```python
from build123d import *

# Parameters (mm, degrees)
F0_R     = 43.2404063775
F1_DEPTH = 77
F1_TAPER = 3
F2_R     = 5
F3_T     = 2.5


with BuildPart() as f1:
    # F0 (on Top) → F1 (new body)
    with BuildSketch(Plane.XY):
        Circle(F0_R)
    extrude(amount=-F1_DEPTH, taper=F1_TAPER)

    # F2
    f2_edges = [f1.edges().sort_by_distance(p)[0] for p in [
        (-39.205007, 0, -77),
    ]]
    fillet(f2_edges, radius=F2_R)

    # F3
    f3_openings = [f1.faces().sort_by_distance(p)[0] for p in [
        (0, 0, 0),
    ]]
    offset(amount=F3_T, openings=f3_openings, kind=Kind.INTERSECTION)


solid = f1.part
```
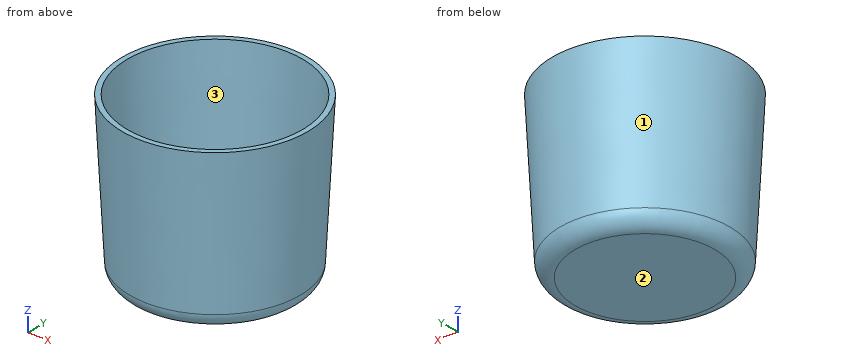
Design review of the part built by this model. Coordinates are the model's own, in mm. Face numbers are marked on the shaded views. Give positions to 0.01 mm unless a question says otherwise; leave off trailing zeros. Loops run counter-clockwise (first coordinate to the right, second up) from the corner with the lowest first, then second, coordinate; pieces in that order, holes last. Notation, with made-up numbers: (-21.5, 62.25) -> (-8.5, 62.25) arc R26 ccw to (-8.5, 92.25) -> close; hole circle Ø6 at (82.25, 81.5). An arc over 180 degrees is marked (long way). One line per item, written item: value.
Q1. For L1, parallel to Z at x = -21.5, y = -22.5; L2, parallel to X at y = -29.5, z = -13; L3, parallel to X at y = -31.5, z = -61.5, list the stretches that pass through material, from the lowest coordinate up.
Numbers:
L1: z = -79.5 to -77
L2: x = -34.06 to -30.68, 30.68 to 34.06
L3: x = -28.56 to -24.68, 24.68 to 28.56
Q2. We need section B-B on z = -52.5. Give the boundary of the cut face in (x, y).
Numbers:
outline: circle Ø85.98 at (0, 0); hole circle Ø80.98 at (0, 0)
Q3. For pin 1 Ø10 at (x, y) = (24.5, 21.5) entering from +Z; pin 2 Ø3 at (y, z) = (-28.5, -54.5) entering from +X; pin 3 Ø1.5 at (x, y) = (19, -10) entering from +Z, all flat-tipped, find the tip position at first contact; note any pin that passes through.
Numbers:
pin 1: stops at z = -75.89
pin 2: stops at x = 33.33
pin 3: stops at z = -77
Q4. We need section C-C on z = -38. Give the boundary of the cut face in (x, y).
Numbers:
outline: circle Ø87.5 at (0, 0); hole circle Ø82.5 at (0, 0)
Q5. Draft analysis for pull direction Y (two halves, no side actions). For the marked faces 1, 2 and 3, state which applies: pulls with the +Y half, pulls with the -Y half, needs draft (parallel to the pull), parting line crosses it, or undercut.
Numbers:
face 1: parting line crosses it
face 2: needs draft
face 3: undercut
Q6. We need section A-A on x = 0. Give the boundary of the cut face in (y, z), and give its area (3 significant figures).
Numbers:
outline: (-45.74, 0) -> (-41.95, -72.39) arc R7.5 ccw to (-34.46, -79.5) -> (34.46, -79.5) arc R7.5 ccw to (41.95, -72.39) -> (45.74, 0) -> (43.24, 0) -> (39.45, -72.26) arc R5 cw to (34.46, -77) -> (-34.46, -77) arc R5 cw to (-39.45, -72.26) -> (-43.24, 0) -> close
area: 582 mm^2
